Geometry: final body of the model. Coordinates: model frame, mm. Face numbers are marked on the shaded views. Give positions to 0.01 mm unless a question says otherwise; leave off trailing zeros. Write each loop counter-clockwise with the first axis right and the second up, starting at its lowest first coordinate (ties: lowest second). Pieces come first, ordered by that corner, then holes.
Q1. Pin query (flat end, axial travel): pin 1 Ø6 at (x, y) = (52.5, -1.5) entering from -Z; pin 2 Ø3 at (x, y) = (32, 4) entering from -Z. Return the tip coordinate at first contact, or that it passes through.
Q2. Section A-A (z = 3.8). State how many separate pieces and enclosed holes the cut face has, plus the area to 3 significant figures.
Q3. Mould query, pull axis Y, two halves, no side actions, for the marked faces 1 and 2. Classes: +Y half, -Y half, draft (parallel to the pull), parting line (faces both ways), or undercut.
Q4. Line query: line 1 (Y direction, x = 56, z = 0.65); line 2 (Y direction, x = 30, z = 0.5); line 3 (Z direction, x = 45, y = 7). Output: solid intervals per line, ascending.
Q5. Section C-C (x = 32). Return the cut outline in (y, z).
from build123d import *

# Parameters (mm, degrees)
F1_DEPTH = 8
F3_W     = 8
F3_H     = 8
F3_R     = 2.4
F4_DEPTH = 1.7
F5_R     = 2.4
F6_DEPTH = 1.7


with BuildPart() as f1:
    # F0 (on Front) → F1 (new body)
    with BuildSketch(Plane.XZ):
        Polygon((-2.4, 3.2333333013), (-4, 3.2333333013), (-4, 0), (4, 0), (4, 3.2333333013), (2.4, 3.2333333013), (2.4, 4.9333333013), (-2.4, 4.9333333013), align=None)
    extrude(amount=F1_DEPTH)

    # F3 (on plane+point) → F4 (cut, through all)
    with BuildSketch(Plane.XY.offset(4.9333333013)):
        with Locations((0, -4)):
            Rectangle(F3_W, F3_H)
        with Locations((0, -4)):
            Circle(F3_R, mode=Mode.SUBTRACT)
    extrude(amount=-F4_DEPTH, mode=Mode.SUBTRACT)

    # F5 (on Top) → F6 (cut)
    with BuildSketch(Plane.XY):
        with Locations((0, -4)):
            Circle(F5_R)
    extrude(amount=F6_DEPTH, mode=Mode.SUBTRACT)

    # F8: F1 across plane


with BuildPart() as f1_1:
    add(f1.part)
    add(f1.part.mirror(Plane.YZ.offset(4)))

    # F9: F1 across plane


with BuildPart() as f1_2:
    add(f1_1.part)
    add(f1_1.part.mirror(Plane.XZ))

    # F11: F1 across plane


with BuildPart() as f1_3:
    add(f1_2.part)
    add(f1_2.part.mirror(Plane.YZ.offset(12)))

    # F12: F1 across face


with BuildPart() as f1_4:
    add(f1_3.part)
    add(f1_3.part.mirror(Plane(origin=(28, 0, 1.6166666507), x_dir=(0, 1, 0), z_dir=(1, 0, 0))))


solid = f1_4.part
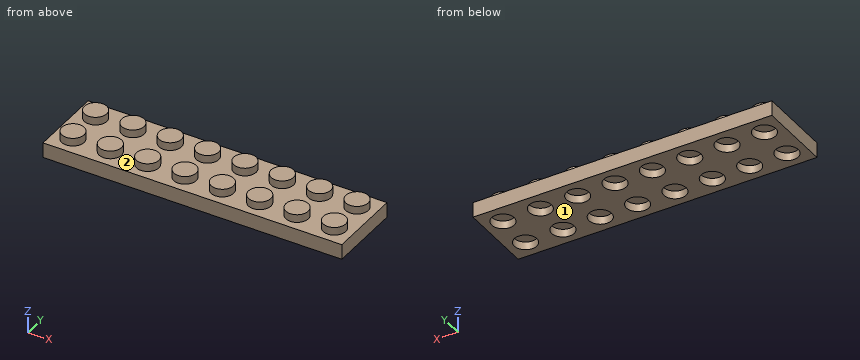
Computed:
1. pin 1: stops at z = 0
1. pin 2: stops at z = 1.7
2. separate pieces: 16
2. enclosed holes: 0
2. area: 290 mm2
3. face 1: draft
3. face 2: undercut
4. line 1: y = -8 to -6.4, -1.6 to 1.6, 6.4 to 8
4. line 2: y = -8 to -5.33, -2.67 to 2.67, 5.33 to 8
4. line 3: z = 0 to 3.23
5. outline: (-8, 0) - (-6.4, 0) - (-6.4, 1.7) - (-1.6, 1.7) - (-1.6, 0) - (1.6, 0) - (1.6, 1.7) - (6.4, 1.7) - (6.4, 0) - (8, 0) - (8, 3.23) - (6.4, 3.23) - (6.4, 4.93) - (1.6, 4.93) - (1.6, 3.23) - (-1.6, 3.23) - (-1.6, 4.93) - (-6.4, 4.93) - (-6.4, 3.23) - (-8, 3.23) - close
